The model under review builds one solid part; all positions refer to its coordinate system, in mm. A direction names the side the tool comes from. Round coordinates to 2 decimals unless told otherwise and drop trailing zeros. Write each loop counter-clockwise with the first axis right and the second up, starting at its lowest first coordinate (ties: lowest second). Pieces come first, ordered by that corner, then holes.
Item 1: Add section C-C (z = 8). Give the boundary of the cut face in (x, y).
Item 2: To check wall thickness, follow L1, parallel to X at y = -22, z = 1.2; L2, parallel to X at y = 23, z = 1.55; L3, parallel to Z at x = 6, y = -5.5. State the ranges of each line that lie inside material, in increasing order.
Item 3: Draft analysis for pull direction Y (two halves, no side actions). For faces 4 (the face through (12, -26, 10)), 5 (the face through (4.1, 15.5, -11.4)), 6 (the face through (-14, -22.5, 6)), state which applies: +Y half, -Y half, draft (parallel to the pull), parting line (faces both ways), or undercut.
Item 4: Clearance check with flat-ended pins moving along their axes: pin 1 Ø4.5 at (x, z) = (-6, 13.5) entering from -Y; pin 2 Ø4.5 at (y, z) = (9, 9) entering from +X; pin 3 Ø8 at (y, z) = (14.5, 8) entering from -X; pin 4 Ø4 at (x, y) = (-22, 9) entering from +Z. State where each tip first meets the part, or that it passes through.
Item 5: Add section D-D (y = 14.5). Give the boundary of the cut face in (x, z), plus the area to 3 significant figures.
Item 6: Add section A-A (x = 12.5). Give the boundary of the cut face in (y, z).
Item 7: Machinability: for faces 1 (the face through (13.5, 7, 11)), 2 (the face through (0, 5, -16)), 3 (the face through (-11, -27, 6)), which of the approach directions +Z, -Z, +X, -X, +Y, -Y give a long, thin tool a straight path to every point of the face, cutting with its end or side? Answer none if there is none.
Item 8: Add section B-B (x = -1.5). Give the boundary of the cut face in (y, z), plus the area to 4 significant figures.
```python
from build123d import *

# Parameters (mm, degrees)
SKETCH_W        = 39
SKETCH_H        = 62
PAD_DEPTH       = 18
SKETCH001_W     = 39
SKETCH001_H     = 21.5
PAD001_DEPTH    = 16
SKETCH002_R     = 3
PAD002_DEPTH    = 13
SKETCH003_W     = 36
SKETCH003_H     = 11
POCKET_DEPTH    = 37.001
POCKET001_DEPTH = 15
SKETCH005_W     = 18
SKETCH005_H     = 0.5
PAD003_DEPTH    = 7
SKETCH006_R     = 2.5
SKETCH006_W     = 6
SKETCH006_H     = 8
PAD004_DEPTH    = 7
SKETCH015_R     = 1.5
POCKET005_DEPTH = 5
SKETCH016_W     = 23
SKETCH016_H     = 10
POCKET006_DEPTH = 49


with BuildPart() as part:
    # Sketch → Pad (new body)
    with BuildSketch(Plane.XY):
        Rectangle(SKETCH_W, SKETCH_H)
    extrude(amount=PAD_DEPTH)

    # Sketch001 (on Face5 of Pad) → Pad001 (join)
    with BuildSketch(Plane(origin=(0, 0, 0), x_dir=(1, 0, 0), z_dir=(0, 0, -1))):
        with Locations((0, -4.75)):
            Rectangle(SKETCH001_W, SKETCH001_H)
    extrude(amount=PAD001_DEPTH)

    # Sketch002 (on Face8 of Pad001) → Pad002 (join)
    with BuildSketch(Plane(origin=(-19.5, 0, 0), x_dir=(0, -1, 0), z_dir=(-1, 0, 0))):
        with Locations((1, -15)):
            Circle(SKETCH002_R)
    extrude(amount=PAD002_DEPTH)

    # Sketch003 (on Face11 of Pad002) → Pocket (cut, through all)
    with BuildSketch(Plane.XZ.offset(6)):
        with Locations((-1.5, -5.5)):
            Rectangle(SKETCH003_W, SKETCH003_H)
    extrude(amount=-POCKET_DEPTH, mode=Mode.SUBTRACT)

    # Sketch004 (on Face6 of Pocket) → Pocket001 (cut)
    with BuildSketch(Plane.XY.offset(18)):
        Polygon((13.5, -17.5), (-14.5, -17.5), (-14.5, 31), (-19.5, 31), (-19.5, -31), (19.5, -31), (19.5, 31), (13.5, 31), align=None)
    extrude(amount=-POCKET001_DEPTH, mode=Mode.SUBTRACT)

    # Sketch005 (on Face15 of Pocket001) → Pad003 (join)
    with BuildSketch(Plane.XZ.offset(17.5)):
        with Locations((0, 15.25)):
            Rectangle(SKETCH005_W, SKETCH005_H)
    extrude(amount=PAD003_DEPTH)

    # Sketch006 (on Face5 of Pad003) → Pad004 (join)
    with BuildSketch(Plane.XY.offset(3)):
        with Locations((12.5, -26)):
            Circle(SKETCH006_R)
        with Locations((-14, -26.5)):
            Rectangle(SKETCH006_W, SKETCH006_H)
    extrude(amount=PAD004_DEPTH)

    # Sketch015 (on Face2 of Pad004) → Pocket005 (cut)
    with BuildSketch(Plane(origin=(0, 0, 0), x_dir=(1, 0, 0), z_dir=(0, 0, -1))):
        with Locations((-8.5, 22)):
            Circle(SKETCH015_R)
        with Locations((8.5, 22)):
            Circle(SKETCH015_R)
        with Locations((-7.5, -23)):
            Circle(SKETCH015_R)
        with Locations((6, -23)):
            Circle(SKETCH015_R)
    extrude(amount=-POCKET005_DEPTH, mode=Mode.SUBTRACT)

    # Sketch016 (on Face1 of Pocket005) → Pocket006 (cut)
    with BuildSketch(Plane(origin=(0, 31, 0), x_dir=(-1, 0, 0), z_dir=(0, 1, 0))):
        with Locations((0.5, 8)):
            Rectangle(SKETCH016_W, SKETCH016_H)
    extrude(amount=-POCKET006_DEPTH, mode=Mode.SUBTRACT)


solid = part.part
```
Numbers:
1. outline: (-17, -30.5) - (-11, -30.5) - (-11, -22.5) - (-17, -22.5) - close; (-14.5, -17.5) - (-12, -17.5) - (-12, 31) - (-14.5, 31) - close; circle Ø5 at (12.5, -26); (11, -17.5) - (13.5, -17.5) - (13.5, 31) - (11, 31) - close
2. L1: x = -19.5 to -10, -7 to 7, 10 to 19.5
2. L2: x = -19.5 to -9, -6 to 4.5, 7.5 to 19.5
2. L3: z = -16 to -11, 0 to 3, 13 to 18
3. face 4: draft
3. face 5: +Y half
3. face 6: undercut
4. pin 1: stops at y = -24.5
4. pin 2: stops at x = 13.5
4. pin 3: stops at x = -14.5
4. pin 4: passes through
5. outline: (-19.5, -16) - (19.5, -16) - (19.5, 3) - (13.5, 3) - (13.5, 18) - (-14.5, 18) - (-14.5, 3) - (-19.5, 3) - (-19.5, 0) - (16.5, 0) - (16.5, -11) - (-19.5, -11) - close; hole (-12, 3) - (11, 3) - (11, 13) - (-12, 13) - close
5. area: 535 mm2
6. outline: (-31, 0) - (31, 0) - (31, 18) - (-17.5, 18) - (-17.5, 3) - (-23.5, 3) - (-23.5, 10) - (-28.5, 10) - (-28.5, 3) - (-31, 3) - close; (-6, -16) - (15.5, -16) - (15.5, -11) - (-6, -11) - close
7. face 1: +Z, +X, +Y
7. face 2: -Z, +X, +Y, -Y
7. face 3: +Z, +Y, -Y
8. outline: (-31, 0) - (31, 0) - (31, 3) - (-31, 3) - close; (-24.5, 15) - (-17.5, 15) - (-17.5, 13) - (31, 13) - (31, 18) - (-17.5, 18) - (-17.5, 15.5) - (-24.5, 15.5) - close; (-6, -16) - (15.5, -16) - (15.5, -11) - (-6, -11) - close
8. area: 539.5 mm2
